from build123d import *

# Parameters (mm, degrees)
SKETCH_1_R      = 1.6
EXTRUDE_1_DEPTH = 3


with BuildPart() as part:
    # 草图1 → 凸台-拉伸1 (new body)
    with BuildSketch(Plane(origin=(0, 0, 0), x_dir=(1, 0, 0), z_dir=(0, 1, 0))):
        with BuildLine():
            Line((-13, -6), (13, -6))
            Line((13, -6), (13, -5.1))
            ThreePointArc((13, -5.1), (11.95, -4.05), (13, -3))
            Line((13, -3), (16.5, -3))
            Line((16.5, -3), (16.5, 3))
            Line((16.5, 3), (13, 3))
            Line((13, 3), (-13, 3))
            Line((-13, 3), (-16.5, 3))
            Line((-16.5, 3), (-16.5, -3))
            Line((-16.5, -3), (-13, -3))
            ThreePointArc((-13, -3), (-12.25753788, -3.30753788), (-11.95, -4.05))
            ThreePointArc((-11.95, -4.05), (-12.25753788, -4.79246212), (-13, -5.1))
            Line((-13, -5.1), (-13, -6))
        make_face()
        with Locations(Location((-4, -3, 0), (0, 0, 270))):
            Circle(SKETCH_1_R, mode=Mode.SUBTRACT)
        with Locations(Location((4, -3, 0), (0, 0, 270))):
            Circle(SKETCH_1_R, mode=Mode.SUBTRACT)
    extrude(amount=EXTRUDE_1_DEPTH)


solid = part.part
Geometry: final body of the model. Coordinates: model frame, mm. A direction names the side the tool comes from. Coordinates: 2 decimals unless noted, no trailing zeros. Order: outer loops, then holes, each group sorted by start corner. A loop starts at its lowest first (then second) coordinate and runs counter-clockwise, first axis right, second up.
(1) Draft query along Z for faces 1 (the face through (13, 1.5, 5.6)), 2 (the face through (3.03, 1.48, 1.73)), 3 (the face through (15, 1, 3)). Return one class per face: pulls with the +Z half, pulls with the -Z half, needs draft (parallel to the pull), parting line crosses it, or undercut.
(2) Section query B-B (z = 2.5). Return the cut outline in (x, y).
(3) First-contact query: pin 1 (1.5 mm diameter, centred on x = 6, z = 3.5, fed in from -Y); pin 2 (0.5 mm diameter, centred on y = 1, z = 5.5, fed in from -X); pin 3 (1 mm diameter, centred on y = 2, z = 5.5, fed in from +X). Flat tips, straight axial feed; report the tip coordinate or a pass-through.
(4) Access query for faces 4 (the face through (0, 0, 1)), 5 (the face through (-15, 1, 3)). Directions: +Z, -Z, +X, -X, +Y, -Y. A direction counts if a zero-diameter tool reaches every point of the face in a straight line with its end or side. Return the directions, or none.
(5) Section query A-A (x = -4). Return the cut outline in (y, z).
(6) Section query C-C (y = 1.7). Return the cut outline in (x, z).
(7) Material intervals for probe 1 along X at (y, z) = (1, 3.25); probe 2 along Z at (x, y) = (-5, 0.75); probe 3 along Z at (x, y) = (15.5, 0.4), sorted ascending.
(8) Section query D-D (z = 5.5). Return the cut outline in (x, y).
Solution:
1. face 1: needs draft
1. face 2: undercut
1. face 3: pulls with the +Z half
2. outline: (-16.5, 0) - (-5.52, 0) - (-5.52, 3) - (-16.5, 3) - close; (-2.48, 0) - (2.48, 0) - (2.48, 3) - (-2.48, 3) - close; (5.52, 0) - (16.5, 0) - (16.5, 3) - (5.52, 3) - close
3. pin 1: stops at y = 0
3. pin 2: stops at x = -13
3. pin 3: stops at x = 13
4. face 4: +Z, -Z, +X, -X, -Y
4. face 5: +Z, -X, +Y, -Y
5. outline: (0, -3) - (3, -3) - (3, 1.4) - (0, 1.4) - close; (0, 4.6) - (3, 4.6) - (3, 6) - (0, 6) - close
6. outline: (-16.5, -3) - (16.5, -3) - (16.5, 3) - (13, 3) arc R1.05 cw to (13, 5.1) - (13, 6) - (-13, 6) - (-13, 5.1) arc R1.05 cw to (-13, 3) - (-16.5, 3) - close; hole circle Ø3.2 at (-4, 3); hole circle Ø3.2 at (4, 3)
7. probe 1: x = -12.32 to -5.58, -2.42 to 2.42, 5.58 to 12.32
7. probe 2: z = -3 to 1.75, 4.25 to 6
7. probe 3: z = -3 to 3
8. outline: (-13, 0) - (13, 0) - (13, 3) - (-13, 3) - close
